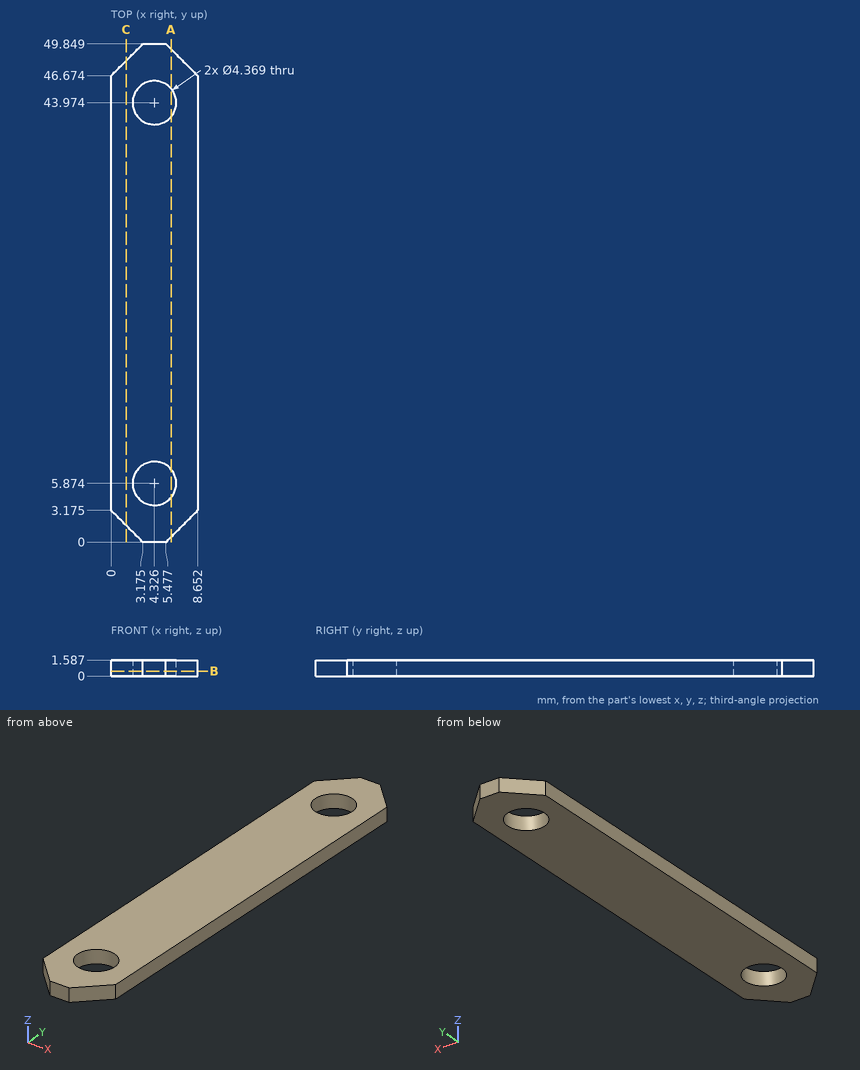
Part print with two shaded views. Sizes in mm from the minimum x, y, z corner. Coordinates: 2 decimals unless noted, no trailing zeros. Loops run counter-clockwise (first coordinate to the right, second up) from the corner with the lowest first, then second, coordinate; pieces in that order, holes last. Notation, with made-up numbers: M -31.5,-37.5 L -2.5,-37.5 A15 cw -2.5,-20.5 Z; hole C 72.25,89 d10. An arc over 180 degrees is marked long. Use CSV: the item, a comma, the result in double quotes. Start each with the question number.
1. Flat gauge pin, fed straight in: pin 1 (5 mm diameter, centred on x = 4.33, y = 43.97, fed in from -Z). Where does the tip first touch, or does it go through?
2. Band-saw the part on C-C, the plane x = 1.5. List the corners of the cut face in (y, z) (1 decimal).
3. Probe probe 1 along Y at (x, z) = (2.5, 0.6) (1 decimal); probe 2 along Y at (x, z) = (5.5, 1.05) (1 decimal); probe 3 along X at (y, z) = (43.5, 1.35) (1 decimal). List the from-to ranges inside material, lowest first. Write a range as [from, to].
4. Band-saw the part on A-A, the plane x = 6. List the corners of the cut face in (y, z).
5. Band-saw the part on B-B, the plane z = 0.5. Give the number of separate pieces and of enclosed holes in the cut face, then the cut area to 3 significant figures.
Entries:
1,pin 1,"stops at z = 0"
2,outline,"M 1.7,0 L 48.2,0 L 48.2,1.6 L 1.7,1.6 Z"
3,probe 1,"y = [0.7, 4.7], [7.1, 42.8], [45.2, 49.2]"
3,probe 2,"y = [0, 4], [7.7, 42.1], [45.8, 49.8]"
3,probe 3,"x = [0, 2.2], [6.5, 8.7]"
4,outline,"M 0.52,0 L 4.47,0 L 4.47,1.59 L 0.52,1.59 Z; M 7.28,0 L 42.57,0 L 42.57,1.59 L 7.28,1.59 Z; M 45.38,0 L 49.33,0 L 49.33,1.59 L 45.38,1.59 Z"
5,separate pieces,"1"
5,enclosed holes,"2"
5,area,"381 mm2"
